The listing builds one solid part. Answer for the finished solid, in the listing's coordinates (mm). A direction names the side the tool comes from. Coordinates: 2 decimals unless noted, no trailing zeros. Order: outer loops, then holes, each group sorted by start corner. A loop starts at its lowest first (then second) coordinate and runs counter-clockwise, first axis right, second up.
```python
from build123d import *

# Parameters (mm, degrees)
F0_W     = 520
F0_H     = 270
F1_DEPTH = 500
F2_W     = 500
F2_H     = 250
F3_DEPTH = 500
F5_DEPTH = 600


with BuildPart() as f1:
    # F0 (on Right) → F1 (new body)
    with BuildSketch(Plane.YZ):
        Rectangle(F0_W, F0_H)
    extrude(amount=-F1_DEPTH)

    # F2 (on face) → F3 (cut)
    with BuildSketch(Plane.YZ):
        Rectangle(F2_W, F2_H)
    extrude(amount=-F3_DEPTH, mode=Mode.SUBTRACT)

    # F4 (on face) → F5 (cut)
    with BuildSketch(Plane.XZ.offset(260)):
        Polygon((-144.166574, 135), (0, -135), (0, 135), align=None)
    extrude(amount=-F5_DEPTH, mode=Mode.SUBTRACT)


solid = f1.part
```
1) A cutting plane is placed at D-D, the plane x = -66.5. Write down the section's boundary in (y, z), plus the area to 3 significant figures.
2) The mould has two halves that part along Z. Classify faces 3 (the flat face through (-317, -3, 125)), 4 (the flat face through (-249, -3, -125)), 5 (the flat face through (-302, -260, -2)), 6 (the flat face through (-141.833, -78.25, 130.63)): released by +Z, released by -Z, zero draft, split by the parting line, or undercut.
3) A cutting plane is placed at A-A, the plane y = -227. Write down the section's boundary in (x, z).
4) For faces 1 (the flat face through (-304, 250, -2)), 2 (the flat face through (-320, -4, 135)), determine the directions among +Z, -Z, +X, -X, +Y, -Y from which every point of the face is accessible in a straight line to the end or side of a thin tool.
5) A cutting plane is placed at B-B, the plane x = -221.5. Write down the section's boundary in (y, z).
6) Straight lines are drawn through the part: probe 1 along Z at (x, y) = (-230, 75.5); probe 2 along Y at (x, z) = (-102, -6); probe 3 along Z at (x, y) = (-112, 74.5). For each, find the intervals that lie inside material, in ascending order.
7) A cutting plane is placed at C-C, the plane z = 17. Write down the section's boundary in (x, y).
Working result:
1. outline: (-260, -135) - (260, -135) - (260, -10.46) - (250, -10.46) - (250, -125) - (-250, -125) - (-250, -10.46) - (-260, -10.46) - close
1. area: 7,490 mm2
2. face 3: undercut
2. face 4: undercut
2. face 5: zero draft
2. face 6: released by +Z
3. outline: (-500, -135) - (0, -135) - (-5.34, -125) - (-500, -125) - close; (-500, 125) - (-138.83, 125) - (-144.17, 135) - (-500, 135) - close
4. face 1: +X, -X
4. face 2: +Z, +X, -X, +Y, -Y
5. outline: (-260, -135) - (260, -135) - (260, 135) - (-260, 135) - close; hole (-250, -125) - (250, -125) - (250, 125) - (-250, 125) - close
6. probe 1: z = -135 to -125, 125 to 135
6. probe 2: y = -260 to -250, 250 to 260
6. probe 3: z = -135 to -125
7. outline: (-500, -260) - (-81.16, -260) - (-81.16, -250) - (-500, -250) - close; (-500, 250) - (-81.16, 250) - (-81.16, 260) - (-500, 260) - close
